from build123d import *

# Parameters (mm, degrees)
SKETCH1_W               = 85.6
SKETCH1_H               = 52.98
BOSS_EXTRUDE1_DEPTH     = 2.4
SKETCH2_R               = 14.1
CUT_EXTRUDE1_DEPTH      = 1.9
SKETCH3_R               = 12.5
CUT_EXTRUDE2_DEPTH      = 1.75
FILLET1_R               = 5
CUT_EXTRUDE3_DEPTH      = 51.39166697
CUT_EXTRUDE3_DEPTH_BACK = 0.5


with BuildPart() as part:
    # Sketch1 → Boss-Extrude1 (new body)
    with BuildSketch(Plane(origin=(0, 0, 0), x_dir=(1, 0, 0), z_dir=(0, 1, 0))):
        Rectangle(SKETCH1_W, SKETCH1_H)
    extrude(amount=BOSS_EXTRUDE1_DEPTH)

    # Sketch2 → Cut-Extrude1 (cut)
    with BuildSketch(Plane(origin=(0, 2.4, 0), x_dir=(1, 0, 0), z_dir=(0, 1, 0))):
        with Locations(Location((-25.8, 9.49, 0), (0, 0, 270))):
            Circle(SKETCH2_R)
        with Locations(Location((0, -9.51, 0), (0, 0, 270))):
            Circle(SKETCH2_R)
        with Locations(Location((25.8, 9.49, 0), (0, 0, 270))):
            Circle(SKETCH2_R)
    extrude(amount=-CUT_EXTRUDE1_DEPTH, mode=Mode.SUBTRACT)

    # Sketch3 → Cut-Extrude2 (cut)
    with BuildSketch(Plane(origin=(0, 0.5, 0), x_dir=(1, 0, 0), z_dir=(0, 1, 0))):
        with Locations(Location((-25.8, 9.49, 0), (0, 0, 270))):
            Circle(SKETCH3_R)
        with Locations(Location((0, -9.51, 0), (0, 0, 270))):
            Circle(SKETCH3_R)
        with Locations(Location((25.8, 9.49, 0), (0, 0, 270))):
            Circle(SKETCH3_R)
    extrude(amount=-CUT_EXTRUDE2_DEPTH, mode=Mode.SUBTRACT)

    # Fillet1
    fillet1_edges = [part.edges().sort_by_distance(p)[0] for p in [
        (42.8, 1.2, 26.49),
        (-42.8, 1.2, 26.49),
        (-42.8, 1.2, -26.49),
        (42.8, 1.2, -26.49),
    ]]
    fillet(fillet1_edges, radius=FILLET1_R)

    # Sketch4 → Cut-Extrude3 (cut, two sides: drawn at the far end of the back side and taken through both)
    with BuildSketch(Plane(origin=(0, 2.4, 0), x_dir=(1, 0, 0), z_dir=(0, 1, 0)).offset(-CUT_EXTRUDE3_DEPTH_BACK)):
        Polygon((-7, 20.49), (-1, 20.49), (-1, 7.49), (1, 7.49), (1, 20.49), (7, 20.49), (7, 22.49), (-7, 22.49), align=None)
    extrude(amount=CUT_EXTRUDE3_DEPTH + CUT_EXTRUDE3_DEPTH_BACK, mode=Mode.SUBTRACT)


solid = part.part
Can you work these out from the model? Positions are in its coordinate system, mm. A direction names the side the tool comes from. Give positions to 0.01 mm unless a question says otherwise; leave off trailing zeros. Loops run counter-clockwise (first coordinate to the right, second up) from the corner with the lowest first, then second, coordinate; pieces in that order, holes last. Notation, with made-up numbers: (61.5, 79.5) - (96.5, 79.5) arc R23 cw to (96.5, 103.5) - close; hole circle Ø3 at (-9, -5). An arc over 180 degrees is marked (long way). One line per item, written item: value.
(1) On a 3-axis mill with a long thin cutter (end or side, diameter ignored), from which of +Z, -Z, +X, -X, +Y, -Y can I reach the whole of each face in a straight line? I mean faces 5 (the face through (13, 0.5, -11)), 6 (the face through (-41.37, 1.22, 24.99)). Say none if no direction works.
Verdict:
face 5: +Y
face 6: +Z, -X, +Y, -Y
(2) If we section it at B-B, the plane y = 0.9: List the corners of the cut face in (x, z) for me, plus the area to 3 significant figures.
Verdict:
outline: (-42.8, -21.49) arc R5 ccw to (-37.8, -26.49) - (37.8, -26.49) arc R5 ccw to (42.8, -21.49) - (42.8, 21.49) arc R5 ccw to (37.8, 26.49) - (-37.8, 26.49) arc R5 ccw to (-42.8, 21.49) - close; hole circle Ø28.2 at (-25.8, -9.49); hole circle Ø28.2 at (0, 9.51); hole circle Ø28.2 at (25.8, -9.49)
area: 2,640 mm^2
(3) If we section it at A-A, the plane x = 0: List the corners of the cut face in (y, z) for me.
Verdict:
outline: (0, -26.49) - (2.4, -26.49) - (2.4, -22.49) - (1.9, -22.49) - (1.9, -7.49) - (2.4, -7.49) - (2.4, -4.59) - (0.5, -4.59) - (0.5, -2.99) - (0, -2.99) - close; (0, 22.01) - (0.5, 22.01) - (0.5, 23.61) - (2.4, 23.61) - (2.4, 26.49) - (0, 26.49) - close
(4) If we section it at D-D, the plane z = -5.5: List the corners of the cut face in (x, y) for me.
Verdict:
outline: (-42.8, 0) - (-37.65, 0) - (-37.65, 0.5) - (-39.32, 0.5) - (-39.32, 2.4) - (-42.8, 2.4) - close; (-13.95, 0) - (13.95, 0) - (13.95, 0.5) - (12.28, 0.5) - (12.28, 2.4) - (-12.28, 2.4) - (-12.28, 0.5) - (-13.95, 0.5) - close; (37.65, 0) - (42.8, 0) - (42.8, 2.4) - (39.32, 2.4) - (39.32, 0.5) - (37.65, 0.5) - close
(5) If we section it at C-C, the plane z = 9.51: List the corners of the cut face in (x, y) for me, plus the area to 3 significant figures.
Verdict:
outline: (-42.8, 0) - (-12.5, 0) - (-12.5, 0.5) - (-14.1, 0.5) - (-14.1, 2.4) - (-42.8, 2.4) - close; (12.5, 0) - (42.8, 0) - (42.8, 2.4) - (14.1, 2.4) - (14.1, 0.5) - (12.5, 0.5) - close
area: 139 mm^2
(6) I'm going to push a flat-ended pin straight in: pin 1 (12 mm diameter, centred on x = -16.5, z = -18.5, fed in from +Y). Where does the tip first touch, or does it pass through?
Verdict:
pin 1: y = 2.4
(7) I need wall thicknesses on line 1 along X through (y, z) = (0.45, -9.49); line 2 along X through (y, z) = (1.75, -9.49); line 3 along Z through (x, y) = (26, 1.85). Which ranges of each line are inside material? Lowest first, please.
Verdict:
line 1: -42.8 to -38.3, -13.3 to 13.3, 38.3 to 42.8
line 2: -42.8 to -39.9, -11.7 to 11.7, 39.9 to 42.8
line 3: -26.49 to -23.59, 4.61 to 26.49
(8) If we mould it in two halves opening along X, with no side actions, what happens to faces 1 (the face through (-5.4, 1.463, 22.535)), 2 (the face through (41.3, 1.22, -25.06)), 3 (the face through (-1, 1, -26.49)), 4 (the face through (-38.3, 0.5, -11.6))? For each: released by +X, released by -X, zero draft, split by the parting line, or undercut.
Verdict:
face 1: undercut
face 2: released by +X
face 3: zero draft
face 4: undercut
